Source: three-view drawing plus pictorial views. Frame: mm from the lowest corner of the part. A direction names the side the tool comes from. Give positions to 0.01 mm unless a question says otherwise; leave off trailing zeros. Write each loop counter-clockwise with the first axis right and the second up, starting at its lowest first coordinate (ties: lowest second). Pieces come first, ordered by that corner, then holes. Notation, with made-up numbers: (-16, 19) -> (3, 19) arc R20 cw to (3, 54) -> close; hole circle Ø6 at (-28, 27). An arc over 180 degrees is marked (long way). Use a Markdown table: item, result. Add a question column.
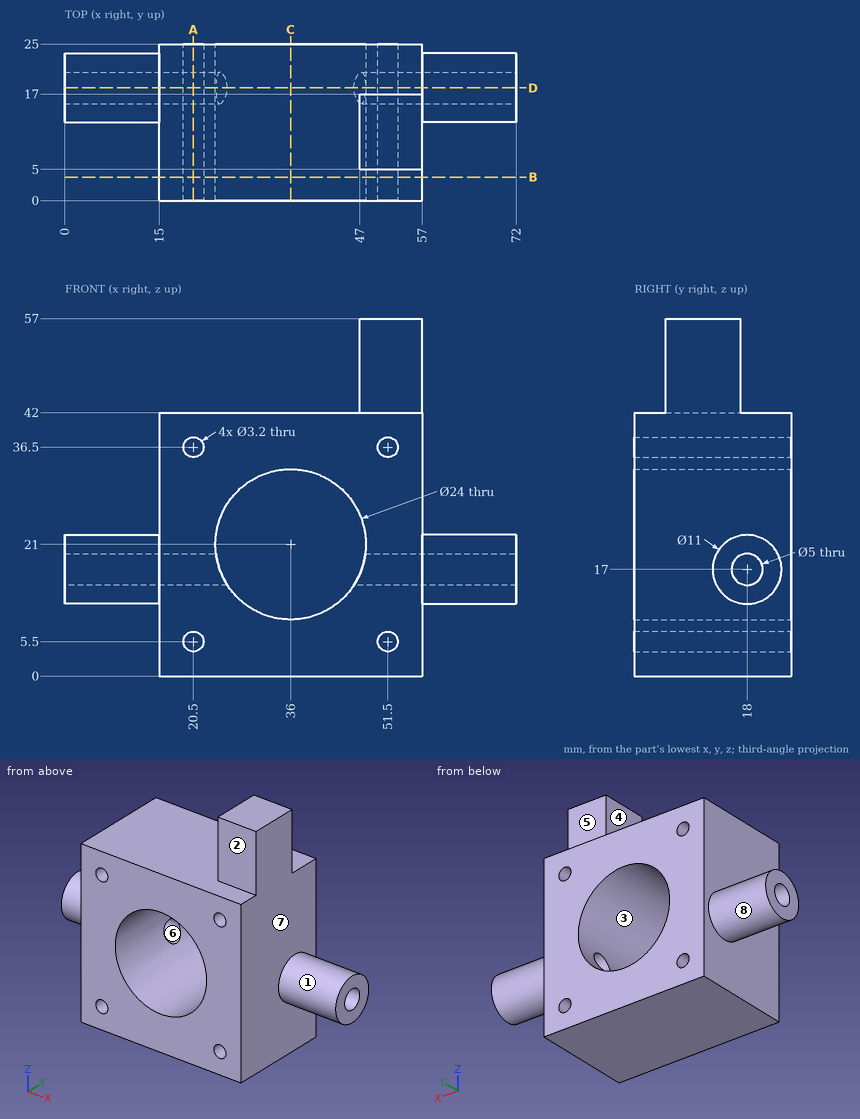
(1) Material intervals for L1, parallel to Z at x = 20.5, y = 8; L2, parallel to Z at x = 51.5, y = 9.5; L3, parallel to Y at x = 19.75, z = 17, sorted ascending.
(2) Cut plane A-A on x = 20.5. Return the cut outline in (y, z), then the cut area to 3 significant figures.
(3) Cut plane B-B on y = 3.75. Return the cut outline in (x, z).
(4) Cut plane C-C on x = 36. Return the cut outline in (y, z), then the cut area to 3 significant figures.
(5) Access query for the marked faces 1, 2, 3, 4 and 5. Directions: +Z, -Z, +X, -X, +Y, -Y. A direction counts if a zero-diameter tool reaches every point of the face in a straight line with its end or side. Return the directions, or none.
(6) Mould query, pull axis Y, two halves, no side actions, for the marked faces 6, 7 and 8. Classes: +Y half, -Y half, draft (parallel to the pull), parting line (faces both ways), or undercut.
(7) Cut plane D-D on y = 18. Return the cut outline in (x, z), then the cut area to 3 significant figures.
(8) First-contact query: pin 1 Ø10 at (x, y) = (22, 7) entering from +Z; pin 2 Ø8 at (x, z) = (50.5, 49) entering from +Y; pin 3 Ø3 at (y, z) = (15.5, 36) entering from +X; pin 4 Ø1.9 at (x, z) = (51.5, 36.5) entering from +Y. Flat tips, straight axial feed; report the tip coordinate or a pass-through.
Output:
| question | item | result |
|---|---|---|
| 1 | L1 | 0 to 3.9, 7.1 to 34.9, 38.1 to 42 |
| 1 | L2 | 0 to 3.9, 7.1 to 34.9, 38.1 to 57 |
| 1 | L3 | 0 to 15.5, 20.5 to 25 |
| 2 | outline | (0, 0) -> (25, 0) -> (25, 3.9) -> (0, 3.9) -> close; (0, 7.1) -> (25, 7.1) -> (25, 34.9) -> (0, 34.9) -> close; (0, 38.1) -> (25, 38.1) -> (25, 42) -> (0, 42) -> close; hole circle Ø5 at (18, 17) |
| 2 | area | 870 mm^2 |
| 3 | outline | (15, 0) -> (57, 0) -> (57, 42) -> (15, 42) -> close; hole circle Ø3.2 at (20.5, 5.5); hole circle Ø3.2 at (20.5, 36.5); hole circle Ø24 at (36, 21); hole circle Ø3.2 at (51.5, 5.5); hole circle Ø3.2 at (51.5, 36.5) |
| 4 | outline | (0, 0) -> (25, 0) -> (25, 9) -> (0, 9) -> close; (0, 33) -> (25, 33) -> (25, 42) -> (0, 42) -> close |
| 4 | area | 450 mm^2 |
| 5 | face 1 | +X |
| 5 | face 2 | +Z, +X, -X, -Y |
| 5 | face 3 | +Y, -Y |
| 5 | face 4 | +Z, -X, +Y, -Y |
| 5 | face 5 | +Z, +X, -X, +Y |
| 6 | face 6 | undercut |
| 6 | face 7 | draft |
| 6 | face 8 | parting line |
| 7 | outline | (0, 11.5) -> (15, 11.5) -> (15, 0) -> (57, 0) -> (57, 11.5) -> (72, 11.5) -> (72, 14.5) -> (46.09, 14.5) arc R12 cw to (25.91, 14.5) -> (0, 14.5) -> close; (0, 19.5) -> (24.09, 19.5) arc R12 cw (long way) to (47.91, 19.5) -> (72, 19.5) -> (72, 22.5) -> (57, 22.5) -> (57, 42) -> (15, 42) -> (15, 22.5) -> (0, 22.5) -> close; hole circle Ø3.2 at (20.5, 5.5); hole circle Ø3.2 at (20.5, 36.5); hole circle Ø3.2 at (51.5, 5.5); hole circle Ø3.2 at (51.5, 36.5) |
| 7 | area | 1,360 mm^2 |
| 8 | pin 1 | z = 42 |
| 8 | pin 2 | y = 17 |
| 8 | pin 3 | x = 57 |
| 8 | pin 4 | through |
